Verification items for the finished model (mm, model axes). A direction names the side the tool comes from. Give positions to 0.01 mm unless a question says otherwise; leave off trailing zeros. Order: outer loops, then holes, each group sorted by start corner. A loop starts at its lowest first (then second) coordinate and runs counter-clockwise, first axis right, second up. Notation, with made-up numbers: (71, -4) -> (113, -4) arc R25 ccw to (113, 33) -> close; hole circle Ø2 at (-39, -11). An arc over 180 degrees is marked (long way). One line per question, with ' | ' between items. Start each with the question number.
Q1. Mould release check, pull along X, two halves, no side actions. Record for faces 3 (the flat face through (7.746, 9.963, 4.056)), 4 (the cylindrical face through (0, -12, 4)), 5 (the flat face through (2.5, 5.2, 8)), 6 (the cylindrical face through (-0.76, 8.05, 6.03)): released by +X, released by -X, zero draft, split by the parting line, or undercut.
Q2. Material ranges on probe 1 along Y at (x, z) = (0, 5.3); probe 2 along Y at (x, z) = (0, 2.2); probe 3 along X at (y, z) = (-6, 1.25), recorded low to high. Write a range as [from, to].
Q3. Section check A-A on y = 0. Record the cut outline in (x, z), plus the area to 3 significant figures.
Q4. Section check D-D on y = -8.5. Record the cut outline in (x, z).
Q5. Go/stop test with flat-tipped pins: pin 1 (11 mm diameter, centred on x = 0, y = 11.47, fed in from +Z); pin 2 (1.5 mm diameter, centred on y = -1, z = 4.5, fed in from +X); pin 3 (1.5 mm diameter, centred on x = -6.36, y = -6.36, fed in from +Z); pin 4 (1.5 mm diameter, centred on y = -5.5, z = 1, fed in from -X). Record where each tip stops, or that it passes through.
Q6. Section check B-B on x = 0. Record the cut outline in (y, z), plus the area to 3 significant figures.
Q7. Access from +Z, -Z, +X, -X, +Y, -Y to the whole of each face (thin tool, end or side, straight path). Record for faces 1 (the cylindrical face through (1.908, 12.069, 2.028)), 2 (the flat face through (2, 10, 4)).
Q8. Section check C-C on z = 7. Record the cut outline in (x, y), plus the area to 3 significant figures.
from build123d import *

# Parameters (mm, degrees)
ESQUISSE1_R             = 12
ESQUISSE1_R_2           = 5.25
BOSS_EXTRU_1_DEPTH      = 8
BOSS_EXTRU_2_DEPTH      = 8
ESQUISSE3_R             = 1.25
ENL_V_MAT_EXTRU_1_DEPTH = 22.401408884
ESQUISSE4_R             = 2
ENL_V_MAT_EXTRU_2_DEPTH = 22.401408884
ESQUISSE5_R             = 3.5
ENL_V_MAT_EXTRU_3_DEPTH = 4


with BuildPart() as part:
    # Esquisse1 → Boss.-Extru.1 (new body)
    with BuildSketch(Plane.XY):
        Circle(ESQUISSE1_R)
        Circle(ESQUISSE1_R_2, mode=Mode.SUBTRACT)
    extrude(amount=BOSS_EXTRU_1_DEPTH)

    # Esquisse2 → Boss.-Extru.2 (add)
    with BuildSketch(Plane.XY.offset(8)):
        with BuildLine():
            Line((-7, 11.468114388), (-8.470537173, 8.5))
            Line((-8.470537173, 8.5), (0, 8.5))
            Line((0, 8.5), (8.470537173, 8.5))
            Line((8.470537173, 8.5), (7, 11.468114388))
            ThreePointArc((7, 11.468114388), (0, 15.8120303), (-7, 11.468114388))
        make_face()
    extrude(amount=-BOSS_EXTRU_2_DEPTH)

    # Esquisse3 → Enlèv. mat.-Extru.1 (cut, through all)
    with BuildSketch(Plane.XY.offset(8)):
        with Locations((-6.363961031, 6.363961031)):
            Circle(ESQUISSE3_R)
        with Locations((6.363961031, 6.363961031)):
            Circle(ESQUISSE3_R)
        with Locations((6.363961031, -6.363961031)):
            Circle(ESQUISSE3_R)
        with Locations((-6.363961031, -6.363961031)):
            Circle(ESQUISSE3_R)
    extrude(amount=-ENL_V_MAT_EXTRU_1_DEPTH, mode=Mode.SUBTRACT)

    # Esquisse4 → Enlèv. mat.-Extru.2 (cut, through all)
    with BuildSketch(Plane.XY.offset(8)):
        with Locations((0, 11.468114388)):
            Circle(ESQUISSE4_R)
    extrude(amount=-ENL_V_MAT_EXTRU_2_DEPTH, mode=Mode.SUBTRACT)

    # Esquisse5 → Enlèv. mat.-Extru.3 (cut)
    with BuildSketch(Plane.XY.offset(8)):
        with Locations((0, 11.468114388)):
            Circle(ESQUISSE5_R)
    extrude(amount=-ENL_V_MAT_EXTRU_3_DEPTH, mode=Mode.SUBTRACT)


solid = part.part
Filled in:
1) face 3: released by +X | face 4: split by the parting line | face 5: zero draft | face 6: undercut
2) probe 1: [-12, -5.25], [5.25, 7.97], [14.97, 15.81] | probe 2: [-12, -5.25], [5.25, 9.47], [13.47, 15.81] | probe 3: [-10.39, -7.56], [-5.17, 5.17], [7.56, 10.39]
3) outline: (-12, 0) -> (-5.25, 0) -> (-5.25, 8) -> (-12, 8) -> close; (5.25, 0) -> (12, 0) -> (12, 8) -> (5.25, 8) -> close | area: 108 mm²
4) outline: (-8.47, 0) -> (8.47, 0) -> (8.47, 8) -> (-8.47, 8) -> close
5) pin 1: z = 8 | pin 2: x = 12 | pin 3: through | pin 4: x = -11.02
6) outline: (-12, 0) -> (-5.25, 0) -> (-5.25, 8) -> (-12, 8) -> close; (5.25, 0) -> (9.47, 0) -> (9.47, 4) -> (7.97, 4) -> (7.97, 8) -> (5.25, 8) -> close; (13.47, 0) -> (15.81, 0) -> (15.81, 8) -> (14.97, 8) -> (14.97, 4) -> (13.47, 4) -> close | area: 94.5 mm²
7) face 1: +Z, -Z | face 2: +Z
8) outline: (-8.47, 8.5) arc R12 ccw (long way) to (8.47, 8.5) -> (7, 11.47) arc R7.81 ccw to (-7, 11.47) -> close; hole circle Ø2.5 at (-6.36, -6.36); hole circle Ø2.5 at (-6.36, 6.36); hole circle Ø10.5 at (0, 0); hole circle Ø7 at (0, 11.47); hole circle Ø2.5 at (6.36, -6.36); hole circle Ø2.5 at (6.36, 6.36) | area: 356 mm²
